from build123d import *

# Parameters (mm, degrees)
CUT_EXTRUDE1_DEPTH              = 1.27
CIRPATTERN1_COUNT               = 6
F_3_4_0_13_DIAMETER_HOLE1_D     = 3.302
F_3_4_0_13_DIAMETER_HOLE1_DEPTH = 15.875
F_3_4_0_13_DIAMETER_HOLE1_TIP   = 0.992020882


with BuildPart() as part:
    # Sketch1 → Revolve1 (revolve)
    with BuildSketch(Plane(origin=(0, 0, 0), x_dir=(0, 0, -1), z_dir=(1, 0, 0))):
        Polygon((0, 12.7), (0, 22.225), (60.452, 22.225), (60.452, 9.525), (79.502, 9.525), (79.502, 0), (57.15, 0), (57.15, 12.7), align=None)
    revolve(axis=Axis((0, 0, 0), (0, 0, -1)))

    # Sketch2 → Cut-Extrude1 (cut)
    with BuildSketch(Plane(origin=(22.225, 0, 0), x_dir=(0, 0, -1), z_dir=(1, 0, 0))):
        with BuildLine():
            Line((7.62, 2.54), (52.832, 2.54))
            ThreePointArc((52.832, 2.54), (55.372, 0), (52.832, -2.54))
            Line((52.832, -2.54), (7.62, -2.54))
            ThreePointArc((7.62, -2.54), (5.08, 0), (7.62, 2.54))
        make_face()
    cut_extrude1 = extrude(amount=-CUT_EXTRUDE1_DEPTH, mode=Mode.SUBTRACT)

    # CirPattern1: Cut-Extrude1 ×6 about axis
    cirpattern1_axis = Axis((0, 0, 0), (0, 0, 1))
    for i in range(1, CIRPATTERN1_COUNT):
        add(cut_extrude1.rotate(cirpattern1_axis, i * 360 / CIRPATTERN1_COUNT), mode=Mode.SUBTRACT)

    # 3/4 (0.13) Diameter Hole1
    with Locations(Plane.XY):
        with Locations((0, 19.05)):
            Hole(F_3_4_0_13_DIAMETER_HOLE1_D / 2, depth=F_3_4_0_13_DIAMETER_HOLE1_DEPTH)
            with Locations((0, 0, -(F_3_4_0_13_DIAMETER_HOLE1_DEPTH + F_3_4_0_13_DIAMETER_HOLE1_TIP / 2))):  # 118° drill point
                Cone(0, F_3_4_0_13_DIAMETER_HOLE1_D / 2, F_3_4_0_13_DIAMETER_HOLE1_TIP, mode=Mode.SUBTRACT)


solid = part.part
Can you work these out from the model? Positions are in its coordinate system, mm. A direction names the side the tool comes from. Coordinates: 2 decimals unless noted, no trailing zeros. Loops run counter-clockwise (first coordinate to the right, second up) from the corner with the lowest first, then second, coordinate; pieces in that order, holes last. Notation, with made-up numbers: (61.5, 4) - (66.5, 4) arc R12 cw to (66.5, 25) - close; hole circle Ø6 at (-18, 37.5). An arc over 180 degrees is marked (long way). Put each result on its own line as item: value. Start each with the question number.
Item 1: If I drill on line 1 along X through (y, z) = (0, -19) (3 decimals); line 2 along Z through (x, y) = (-14, 3.5); line 3 along Y through (x, z) = (-3, -51), over which ranges is the centre line in solid material (lowest first)?
Item 2: Suppose I cut it at B-B (y = 0). Please give me the cut outline in (x, z) (3 decimals).
Item 3: Suppose I cut it at C-C (x = 5). Please give me the cut outline in (y, z).
Item 4: Suppose I cut it at D-D (y = -6.5). Please give me the cut outline in (x, z), and give its area (3 significant figures).
Item 5: Which directions (+Z, -Z, +X, -X, +Y, -Y) give clear straight access to the entire face, cutting with the end or side of a thin tool? Please do faces 4 (the face through (10.85, 18.68, -5.08)), 5 (the face through (20.955, 0, -31)), 6 (the face through (-5.796, -7.559, -70.11)).
Item 6: If we mould it in two halves opening along Z, with no side actions, what happens to faces 1 (the face through (-10.75, -18.73, -55.37)), 2 (the face through (0, 0, -57.15)), 3 (the face through (0, 0, -79.502))? For each: +Z half, -Z half, draft (parallel to the pull), parting line (faces both ways), or undercut.
Item 7: Suppose I cut it at A-A (z = -18). Please give me the cut outline in (x, y) (3 decimals).
Item 8: For pin 1 (10 mm diameter, centred on y = 5.5, z = -15.5, fed in from -X); pin 2 (8 mm diameter, centred on y = 0, z = -67.5, fed in from -X) (3 decimals); pin 3 (12 mm diameter, centred on x = -12.5, y = 0.5, fed in from +Z); pin 4 (4 mm diameter, centred on y = 10, z = -8.5, fed in from +X), each with a flat end and sliding along its axis, tell me the tip position at first contact or that it passes through.
Here are the results:
1. line 1: -20.955 to -12.7, 12.7 to 20.955
1. line 2: -60.45 to 0
1. line 3: -22.02 to -12.34, 12.34 to 22.02
2. outline: (-22.225, -60.452) - (-9.525, -60.452) - (-9.525, -79.502) - (9.525, -79.502) - (9.525, -60.452) - (22.225, -60.452) - (22.225, -55.372) - (20.955, -55.372) - (20.955, -5.08) - (22.225, -5.08) - (22.225, 0) - (12.7, 0) - (12.7, -57.15) - (-12.7, -57.15) - (-12.7, 0) - (-22.225, 0) - (-22.225, -5.08) - (-20.955, -5.08) - (-20.955, -55.372) - (-22.225, -55.372) - close
3. outline: (-21.66, -60.45) - (-8.11, -60.45) - (-8.11, -79.5) - (8.11, -79.5) - (8.11, -60.45) - (21.66, -60.45) - (21.66, 0) - (11.67, 0) - (11.67, -57.15) - (-11.67, -57.15) - (-11.67, 0) - (-21.66, 0) - close
4. outline: (-21.25, -60.45) - (-6.96, -60.45) - (-6.96, -79.5) - (6.96, -79.5) - (6.96, -60.45) - (21.25, -60.45) - (21.25, 0) - (10.91, 0) - (10.91, -57.15) - (-10.91, -57.15) - (-10.91, 0) - (-21.25, 0) - close
4. area: 1,590 mm²
5. face 4: none
5. face 5: +X
5. face 6: -Z
6. face 1: undercut
6. face 2: +Z half
6. face 3: -Z half
7. outline: (-22.079, -2.54) arc R22.225 ccw to (-13.239, -17.851) - (-12.677, -16.878) - (-8.278, -19.418) - (-8.84, -20.391) arc R22.225 ccw to (8.84, -20.391) - (8.278, -19.418) - (12.677, -16.878) - (13.239, -17.851) arc R22.225 ccw to (22.079, -2.54) - (20.955, -2.54) - (20.955, 2.54) - (22.079, 2.54) arc R22.225 ccw to (13.239, 17.851) - (12.677, 16.878) - (8.278, 19.418) - (8.84, 20.391) arc R22.225 ccw to (-8.84, 20.391) - (-8.278, 19.418) - (-12.677, 16.878) - (-13.239, 17.851) arc R22.225 ccw to (-22.079, 2.54) - (-20.955, 2.54) - (-20.955, -2.54) - close; hole circle Ø25.4 at (0, 0)
8. pin 1: x = -22.08
8. pin 2: x = -9.525
8. pin 3: z = 0
8. pin 4: x = 20.74
